The listing builds one solid part. Answer for the finished solid, in the listing's coordinates (mm). Face numbers are marked on the shaded views. A direction names the side the tool comes from. Round coordinates to 2 decimals unless told otherwise and drop trailing zeros. Write each loop counter-clockwise with the first axis right and the second up, starting at its lowest first coordinate (ties: lowest second). Pieces come first, ordered by that corner, then holes.
(1) A cutting plane is placed at B-B, the plane z = -16.5. Give the vertices of the cut face in (x, y), and give its area (3 significant figures).
(2) For the marked faces 1 and 2, determine the directions among +Z, -Z, +X, -X, +Y, -Y from which every point of the face is accessible in a straight line to the end or side of a thin tool.
(3) A cutting plane is placed at A-A, the plane z = 13. Give the vertices of the cut face in (x, y).
(4) Find the intervals of material crossed by probe 1 along X at (y, z) = (6.25, 12.5); probe 2 along X at (y, z) = (1.75, 26.5); probe 3 along Z at (x, y) = (-19, 4.25), in increasing order.
(5) The mould has two halves that part along X. Classify the marked faces 3 and 4: +X half, -X half, draft (parallel to the pull), parting line (faces both ways), or undercut.
(6) Each of these flat-tipped pins is pushed along its axis until it touches: pin 1 Ø1.9 at (y, z) = (4.5, 28.5) entering from -X; pin 2 Ø3 at (x, y) = (-13, 4.5) entering from +Z; pin 3 Ø3 at (y, z) = (2, 29) entering from +X. Where does it stop, or does it pass through?
(7) A cutting plane is placed at D-D, the plane y = 4. Give the number of separate pieces and of enclosed holes in the cut face, and give its area (3 significant figures).
(8) A cutting plane is placed at C-C, the plane x = -16. Give the vertices of the cut face in (y, z).
from build123d import *

# Parameters (mm, degrees)
ESQUISSE2_W             = 86.602540378
ESQUISSE2_H             = 50
BOSS_EXTRU_1_DEPTH      = 6.35
SKETCH1_R               = 4.7625
CUT_EXTRUDE1_DEPTH      = 6.35
ESQUISSE3_W             = 15
ESQUISSE3_H             = 6.35
BOSS_EXTRU_2_DEPTH      = 6.35
ESQUISSE4_W             = 6.35
ESQUISSE4_H             = 20
ENL_V_MAT_EXTRU_1_DEPTH = 6.35


with BuildPart() as part:
    # Esquisse2 → Boss.-Extru.1 (new body)
    with BuildSketch(Plane(origin=(0, 0, 0), x_dir=(1, 0, 0), z_dir=(0, 1, 0))):
        Rectangle(ESQUISSE2_W, ESQUISSE2_H)
    extrude(amount=BOSS_EXTRU_1_DEPTH)

    # Sketch1 → Cut-Extrude1 (cut)
    with BuildSketch(Plane(origin=(0, 6.35, 0), x_dir=(1, 0, 0), z_dir=(0, 1, 0))):
        with Locations(Location((0, 16.5, 0), (0, 0, 270))):
            Circle(SKETCH1_R)
    extrude(amount=-CUT_EXTRUDE1_DEPTH, mode=Mode.SUBTRACT)

    # Esquisse3 → Boss.-Extru.2 (add)
    with BuildSketch(Plane.XY.offset(25)):
        with Locations((30.801270189, 3.175)):
            Rectangle(ESQUISSE3_W, ESQUISSE3_H)
        with Locations((-30.801270189, 3.175)):
            Rectangle(ESQUISSE3_W, ESQUISSE3_H)
        with Locations((0, 3.175)):
            Rectangle(ESQUISSE3_W, ESQUISSE3_H)
    extrude(amount=BOSS_EXTRU_2_DEPTH)

    # Esquisse4 → Enlèv. mat.-Extru.1 (cut)
    with BuildSketch(Plane.XZ):
        with Locations((18.175, 5)):
            Rectangle(ESQUISSE4_W, ESQUISSE4_H)
        with Locations((-18.175, 5)):
            Rectangle(ESQUISSE4_W, ESQUISSE4_H)
    extrude(amount=-ENL_V_MAT_EXTRU_1_DEPTH, mode=Mode.SUBTRACT)


solid = part.part
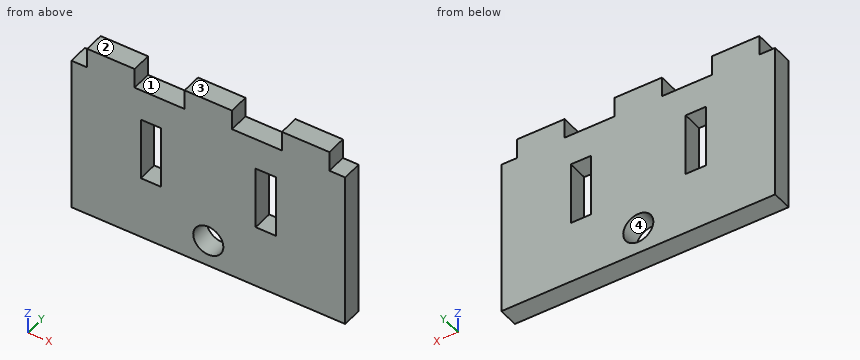
Solutions:
1. outline: (-43.3, 0) - (-4.76, 0) - (-4.76, 6.35) - (-43.3, 6.35) - close; (4.76, 0) - (43.3, 0) - (43.3, 6.35) - (4.76, 6.35) - close
1. area: 489 mm2
2. face 1: +Z, +Y, -Y
2. face 2: +Z, +X, -X, +Y, -Y
3. outline: (-43.3, 0) - (-21.35, 0) - (-21.35, 6.35) - (-43.3, 6.35) - close; (-15, 0) - (15, 0) - (15, 6.35) - (-15, 6.35) - close; (21.35, 0) - (43.3, 0) - (43.3, 6.35) - (21.35, 6.35) - close
4. probe 1: x = -43.3 to -21.35, -15 to 15, 21.35 to 43.3
4. probe 2: x = -38.3 to -23.3, -7.5 to 7.5, 23.3 to 38.3
4. probe 3: z = -25 to -5, 15 to 25
5. face 3: draft
5. face 4: undercut
6. pin 1: stops at x = -38.3
6. pin 2: stops at z = 25
6. pin 3: stops at x = 38.3
7. separate pieces: 1
7. enclosed holes: 3
7. area: 4,290 mm2
8. outline: (0, -25) - (6.35, -25) - (6.35, -5) - (0, -5) - close; (0, 15) - (6.35, 15) - (6.35, 25) - (0, 25) - close
